The listing builds one solid part. Answer for the finished solid, in the listing's coordinates (mm). A direction names the side the tool comes from. Round coordinates to 2 decimals unless told otherwise and drop trailing zeros. Order: outer loops, then holes, each group sorted by start corner. A loop starts at its lowest first (then second) coordinate and runs counter-clockwise, first axis right, second up. Notation, with made-up numbers: (67.25, 58.5) - (79.25, 58.5) arc R26 cw to (79.25, 76.5) - close; hole circle Ø7 at (-37, 36). An arc over 180 degrees is marked (long way). Write item = value, one per line.
from build123d import *

# Parameters (mm, degrees)
SKETCH_1_R          = 40
EXTRUDE_1_DEPTH     = 12
SKETCH_8_R          = 45
EXTRUDE_3_DEPTH     = 2
SKETCH_2_R          = 7.5
CUT_EXTRUDE_1_DEPTH = 66.161338231
HOLE_WIZARD_M32_D   = 3.4
CUT_EXTRUDE_2_DEPTH = 66.161338231
HOLE_WIZARD_M33_D   = 3.4
SKETCH_17_R         = 42.242904023
CUT_EXTRUDE_3_DEPTH = 12
SKETCH_18_R         = 27
CUT_EXTRUDE_4_DEPTH = 64.671029519
FILLET_1_R          = 5


with BuildPart() as part:
    # Эскиз1 → Бобышка-Вытянуть1 (new body)
    with BuildSketch(Plane.XY):
        Circle(SKETCH_1_R)
    extrude(amount=EXTRUDE_1_DEPTH)

    # Эскиз8 → Бобышка-Вытянуть3 (add)
    with BuildSketch(Plane.XY.offset(12)):
        Circle(SKETCH_8_R)
    extrude(amount=EXTRUDE_3_DEPTH)

    # Эскиз2 → Вырез-Вытянуть1 (cut, through all)
    with BuildSketch(Plane(origin=(0, 0, 14), x_dir=(-1, 0, 0), z_dir=(0, 0, -1))):
        Circle(SKETCH_2_R)
    extrude(amount=CUT_EXTRUDE_1_DEPTH, mode=Mode.SUBTRACT)

    # Отверстие с зазором M32 (through all)
    with Locations(Plane.XY.offset(14)):
        with Locations((6.25, 10.825317547), (-12.5, 0), (6.25, -10.825317547)):
            Hole(HOLE_WIZARD_M32_D / 2)

    # Эскиз10 → Вырез-Вытянуть2 (cut, through all)
    with BuildSketch(Plane(origin=(0, 0, 0), x_dir=(-1, 0, 0), z_dir=(0, 0, -1))):
        with BuildLine():
            ThreePointArc((32.475952642, -18.75), (28.632685902, -4.40673326), (14.289419162, -8.25))
            ThreePointArc((14.289419162, -8.25), (8.25, -14.289419162), (0, -16.5))
            ThreePointArc((0, -16.5), (-10.5, -27), (0, -37.5))
            ThreePointArc((0, -37.5), (18.75, -32.475952642), (32.475952642, -18.75))
        make_face()
        with BuildLine():
            ThreePointArc((32.475952642, 18.75), (18.75, 32.475952642), (0, 37.5))
            ThreePointArc((0, 37.5), (-10.5, 27), (0, 16.5))
            ThreePointArc((0, 16.5), (8.25, 14.289419162), (14.289419162, 8.25))
            ThreePointArc((14.289419162, 8.25), (28.632685902, 4.40673326), (32.475952642, 18.75))
        make_face()
        with BuildLine():
            ThreePointArc((-32.475952642, -18.75), (-18.132685902, -22.59326674), (-14.289419162, -8.25))
            ThreePointArc((-14.289419162, -8.25), (-16.5, 0), (-14.289419162, 8.25))
            ThreePointArc((-14.289419162, 8.25), (-18.132685902, 22.59326674), (-32.475952642, 18.75))
            ThreePointArc((-32.475952642, 18.75), (-37.5, 0), (-32.475952642, -18.75))
        make_face()
    extrude(amount=-CUT_EXTRUDE_2_DEPTH, mode=Mode.SUBTRACT)

    # Отверстие с зазором M33 (through all)
    with Locations(Plane(origin=(0, 0, 0), x_dir=(-1, 0, 0), z_dir=(0, 0, -1))):
        with Locations((-17.5, 30.310889132), (35, 0), (-17.5, -30.310889132)):
            Hole(HOLE_WIZARD_M33_D / 2)

    # Эскиз17 → Вырез-Вытянуть3 (cut)
    with BuildSketch(Plane(origin=(0, 0, 0), x_dir=(-1, 0, 0), z_dir=(0, 0, -1))):
        Circle(SKETCH_17_R)
    extrude(amount=-CUT_EXTRUDE_3_DEPTH, mode=Mode.SUBTRACT)

    # Эскиз18 → Вырез-Вытянуть4 (cut, through all)
    with BuildSketch(Plane(origin=(0, 0, 12), x_dir=(-1, 0, 0), z_dir=(0, 0, -1))):
        Circle(SKETCH_18_R)
    extrude(amount=-CUT_EXTRUDE_4_DEPTH, mode=Mode.SUBTRACT)

    # Скругление1
    fillet_1_edges = [part.edges().sort_by_distance(p)[0] for p in [
        (16.464754658, 21.398875065, 13),
        (10.29959209, 24.958333333, 13),
        (-26.764346748, 3.559458268, 13),
        (-26.764346748, -3.559458268, 13),
        (10.29959209, -24.958333333, 13),
        (16.464754658, -21.398875065, 13),
    ]]
    fillet(fillet_1_edges, radius=FILLET_1_R)


solid = part.part
Q1. For faces 1 (the face through (-30, 4, 12)), 2 (the face through (-18.988, 32.338, 12.986)), determine the directions among +Z, -Z, +X, -X, +Y, -Y from which every point of the face is accessible in a straight line to the end or side of a thin tool.
Model answer:
face_1 = -Z, +X, -X, +Y, -Y
face_2 = +Z, -Z
Q2. Section C-C on z = 12.4 is taken. Count the separate pieces of the cut face and the enclosed holes in it, then the cut area to 3 significant figures.
Model answer:
separate_pieces = 1
enclosed_holes = 4
area = 2,410 mm^2
Q3. Determine the mould class of faces 3 (the face through (20.765, -39.923, 12.986)), 4 (the face through (-30, 4, 14)), 5 (the face through (7.097, 34.739, 12.986)) for opening direction X: released by +X, released by -X, zero draft, split by the parting line, or undercut.
Model answer:
face_3 = split by the parting line
face_4 = zero draft
face_5 = undercut
Q4. Find the intervals of material crossed by line 1 (Y direction, x = -31.5, z = 12.2); line 2 (Y direction, x = 17.5, z = 12.65); line 3 (X direction, y = 30, z = 13.3), in increasing order. Write a range as from..to.
Model answer:
line_1 = -32.14..-20.35, -6.84..6.84, 20.35..32.14
line_2 = -41.46..-32.01, -28.61..-22.5, 22.5..28.61, 32.01..41.46
line_3 = -33.54..-22.5, 10.06..15.83, 19.17..33.54
Q5. Section A-A on y = 21 is taken. Determine the outline of the cut face in (x, z).
Model answer:
outline = (-39.8, 12) - (-31.07, 12) - (-31.07, 14) - (-39.8, 14) - close; (30.73, 12) - (39.8, 12) - (39.8, 14) - (30.73, 14) - close
Q6. Section B-B on x = -9 is taken. Determine the outline of the cut face in (y, z).
Model answer:
outline = (-44.09, 12) - (-36.4, 12) - (-36.4, 14) - (-44.09, 14) - close; (36.4, 12) - (44.09, 12) - (44.09, 14) - (36.4, 14) - close
Q7. Flat-ended cylindrical pins translate along their axes: P1, Ø2, axis at x = 17.5, y = -30.31, coming from the +Z side; P2, Ø1, axis at y = -6.5, z = 12.5, coming from the +X side. Find the tip coordinate at first contact, or state that the pin passes through.
Model answer:
P1 = through
P2 = 44.6
